Geometry: final body of the model. Coordinates: model frame, mm. A direction names the side the tool comes from. Coordinates: 2 decimals unless noted, no trailing zeros. Order: outer loops, then holes, each group sorted by start corner. A loop starts at its lowest first (then second) coordinate and runs counter-clockwise, first axis right, second up. Notation, with made-up numbers: (37.5, -14) -> (72.5, -14) arc R26 cw to (72.5, 14) -> close; hole circle Ø9 at (2, -31.75). An arc over 180 degrees is marked (long way). Answer in a Markdown table with one row per item. Add a question column.
1) Section query B-B on x = 12. Return the cut outline in (y, z), then the cut area to 3 significant figures.
2) Contact query for flat-ended pins moving along their axis: P1, Ø2, axis at y = -11, z = 7.5, coming from the -X side; P2, Ø2, axis at x = -1, z = 8.5, coming from the +Y side; P3, Ø3, axis at x = 0, z = 6.35, coming from the +Y side; P4, Ø2, axis at x = -0.5, z = 6.5, coming from the -Y side. Output: stop coordinate, or through.
3) Section query A-A on y = 7.5. Return the cut outline in (x, z).
4) Pull-direction query (X, two-part tool) for faces 1 (the face through (-3.772, -16.985, 6.261)), 2 (the face through (3.302, -11, 6)), 3 (the face through (0, -9, 0)); classes: +X half, -X half, draft (parallel to the pull), parting line (faces both ways), or undercut.
5) Section query D-D on x = 2.5. Return the cut outline in (y, z), then the cut area to 3 significant figures.
6) Set-up query: faces 4 (the face through (0, -9, 8)), 5 (the face through (-3.302, -11, 6)), 6 (the face through (0, -9, 12.7)), 7 (the face through (-3, -11.938, 9)). Return all of +Z, -Z, +X, -X, +Y, -Y with unobstructed straight access to the full face (end or side cutting, diameter ignored); none if empty.
7) Ray query, line 1 (Y direction, x = 0, z = 10); line 2 (Y direction, x = 5.5, z = 4.75); line 3 (Y direction, x = -4.5, z = 1.5). Return the intervals inside material, ascending. Write a range as from..to.
8) Section query C-C on z = 1.5. Return the cut outline in (x, y).
```python
from build123d import *

# Parameters (mm, degrees)
F0_R     = 17.399
F1_DEPTH = 12.7
F2_R     = 1.651
F3_DEPTH = 3.81
F5_DEPTH = 2.54
F6_R     = 3.81
F7_DEPTH = 25.528


with BuildPart() as f1:
    # F0 (on Top) → F1 (new body)
    with BuildSketch(Plane.XY):
        Circle(F0_R)
        with BuildLine():
            ThreePointArc((10.845681, -11.938), (0, -16.129), (-10.845681, -11.938))
            Line((-10.845681, -11.938), (10.845681, -11.938))
        make_face(mode=Mode.SUBTRACT)
        with BuildLine():
            Line((13.931269, -8.128), (-13.931269, -8.128))
            ThreePointArc((-13.931269, -8.128), (0, 16.129), (13.931269, -8.128))
        make_face(mode=Mode.SUBTRACT)
    extrude(amount=F1_DEPTH)

    # F2 (on face) → F3 (cut, through all)
    with BuildSketch(Plane(origin=(0, -8.128, 0), x_dir=(-1, 0, 0), z_dir=(0, 1, 0))):
        with Locations((0, 6.35)):
            Circle(F2_R)
    extrude(amount=-F3_DEPTH, mode=Mode.SUBTRACT)

    # F4 (on face) → F5 (cut)
    with BuildSketch(Plane.XZ.offset(11.938)):
        Polygon((3.302, 4.443589), (3.302, 8.256411), (0, 10.162821), (-3.302, 8.256411), (-3.302, 4.443589), (0, 2.537179), align=None)
    extrude(amount=-F5_DEPTH, mode=Mode.SUBTRACT)

    # F6 (on face) → F7 (cut, through all)
    with BuildSketch(Plane(origin=(0, -8.128, 0), x_dir=(-1, 0, 0), z_dir=(0, 1, 0))):
        with Locations((0, 6.35)):
            Circle(F6_R)
    extrude(amount=F7_DEPTH, mode=Mode.SUBTRACT)


solid = f1.part
```
Result:
| question | item | result |
|---|---|---|
| 1 | outline | (-12.6, 0) -> (-8.13, 0) -> (-8.13, 12.7) -> (-12.6, 12.7) -> close; (10.78, 0) -> (12.6, 0) -> (12.6, 12.7) -> (10.78, 12.7) -> close |
| 1 | area | 79.9 mm2 |
| 2 | P1 | x = -14.24 |
| 2 | P2 | y = -8.13 |
| 2 | P3 | y = -16.06 |
| 2 | P4 | y = -17.4 |
| 3 | outline | (-15.7, 0) -> (-14.28, 0) -> (-14.28, 12.7) -> (-15.7, 12.7) -> close; (14.28, 0) -> (15.7, 0) -> (15.7, 12.7) -> (14.28, 12.7) -> close |
| 4 | face 1 | parting line |
| 4 | face 2 | undercut |
| 4 | face 3 | draft |
| 5 | outline | (-17.22, 0) -> (-15.93, 0) -> (-15.93, 12.7) -> (-17.22, 12.7) -> close; (-11.94, 0) -> (-8.13, 0) -> (-8.13, 12.7) -> (-11.94, 12.7) -> (-11.94, 8.72) -> (-9.4, 8.72) -> (-9.4, 3.98) -> (-11.94, 3.98) -> close; (15.93, 0) -> (17.22, 0) -> (17.22, 3.47) -> (15.93, 3.47) -> close; (15.93, 9.23) -> (17.22, 9.23) -> (17.22, 12.7) -> (15.93, 12.7) -> close |
| 5 | area | 61.6 mm2 |
| 6 | face 4 | +Y |
| 6 | face 5 | none |
| 6 | face 6 | +Z, +X, -X, +Y, -Y |
| 6 | face 7 | +Z, -Z |
| 7 | line 1 | -17.4..-16.13, -9.4..-8.13 |
| 7 | line 2 | -16.51..-15.16, -11.94..-8.13, 15.16..16.51 |
| 7 | line 3 | -16.81..-15.49, -11.94..-8.13, 15.49..16.81 |
| 8 | outline | circle Ø34.8 at (0, 0); hole (-13.93, -8.13) -> (13.93, -8.13) arc R16.13 ccw (long way) to start; hole (-10.85, -11.94) arc R16.13 ccw to (10.85, -11.94) -> close |
